from build123d import *

# Parameters (mm, degrees)
F0_R     = 2.5
F1_DEPTH = 5


with BuildPart() as f1:
    # F0 (on Front) → F1 (new body)
    with BuildSketch(Plane.XZ):
        with BuildLine():
            ThreePointArc((0, -4.25), (3.005204, -3.005204), (4.25, 0))
            ThreePointArc((4.25, 0), (3.005204, 3.005204), (0, 4.25))
            ThreePointArc((0, 4.25), (-4.25, 0), (0, -4.25))
        make_face()
        Circle(F0_R, mode=Mode.SUBTRACT)
        with BuildLine():
            ThreePointArc((30.75, 0), (29.505204, 3.005204), (26.5, 4.25))
            ThreePointArc((26.5, 4.25), (22.25, 0), (26.5, -4.25))
            ThreePointArc((26.5, -4.25), (29.505204, -3.005204), (30.75, 0))
        make_face()
        with Locations((26.5, 0)):
            Circle(F0_R, mode=Mode.SUBTRACT)
        with BuildLine():
            ThreePointArc((0, 4.25), (3.005204, 3.005204), (4.25, 0))
            ThreePointArc((4.25, 0), (3.005204, -3.005204), (0, -4.25))
            Line((0, -4.25), (26.5, -4.25))
            ThreePointArc((26.5, -4.25), (22.25, 0), (26.5, 4.25))
            Line((26.5, 4.25), (0, 4.25))
        make_face()
    extrude(amount=F1_DEPTH)


solid = f1.part
For this review, take the finished solid that the model builds, in its own axes (mm). Round coordinates to 2 decimals unless told otherwise and drop trailing zeros. Loops run counter-clockwise (first coordinate to the right, second up) from the corner with the lowest first, then second, coordinate; pieces in that order, holes last. Notation, with made-up numbers: (64, 41.5) - (119, 41.5) arc R10 ccw to (119, 58.5) - close; hole circle Ø1 at (-10, 50.5). An arc over 180 degrees is marked (long way). Answer as CSV lines item,"result".
(1) Insertion check: P1, Ø1.5, axis at y = -2, z = -2, coming from the +X side; P2, Ø1, axis at y = -3, z = 2.5, coming from the -X side. Each pin has a flat end and moves straight along its axis. Give the tip position at first contact, or say it passes through.
Checked values:
P1,"stops at x = 30.56"
P2,"stops at x = -3.75"
(2) Consider section C-C on y = -4.35. Give the boundary of the cut face in (x, z), then the cut area to 3 significant figures.
Checked values:
outline,"(0, -4.25) - (26.5, -4.25) arc R4.25 ccw to (30.75, 0) arc R4.25 ccw to (26.5, 4.25) - (0, 4.25) arc R4.25 ccw to start; hole circle Ø5 at (0, 0); hole circle Ø5 at (26.5, 0)"
area,"243 mm2"
(3) Consider section D-D on z = -3. Give the boundary of the cut face in (x, y), then the cut area to 3 significant figures.
Checked values:
outline,"(-3.01, -5) - (29.51, -5) - (29.51, 0) - (-3.01, 0) - close"
area,"163 mm2"
(4) Consider section A-A on z = 2. Give the boundary of the cut face in (x, y).
Checked values:
outline,"(-3.75, -5) - (-1.5, -5) - (-1.5, 0) - (-3.75, 0) - close; (1.5, -5) - (25, -5) - (25, 0) - (1.5, 0) - close; (28, -5) - (30.25, -5) - (30.25, 0) - (28, 0) - close"
(5) Mouldability with a two-part tool opening along X and no side actions: class faces 1 (the face through (24, -2, 0)), 2 (the face through (-4.25, -2.46, 0.09)), 3 (the face through (13, -2, -4.25)) as +X half, -X half, draft (parallel to the pull), parting line (faces both ways), or undercut.
Checked values:
face 1,"undercut"
face 2,"-X half"
face 3,"draft"
(6) Consider section B-B on x = 28.5. Give the boundary of the cut face in (y, z).
Checked values:
outline,"(-5, -3.75) - (0, -3.75) - (0, -1.5) - (-5, -1.5) - close; (-5, 1.5) - (0, 1.5) - (0, 3.75) - (-5, 3.75) - close"
(7) Wall thickness on line 1 (X direction, y = -3.05, z = -0.75); line 2 (X direction, y = -2.75, z = 1.5); line 3 (Z direction, x = 26.5, y = -1.6): over which ranges is each line inside the solid? List them lowest first.
Checked values:
line 1,"x = -4.18 to -2.38, 2.38 to 24.12, 28.88 to 30.68"
line 2,"x = -3.98 to -2, 2 to 24.5, 28.5 to 30.48"
line 3,"z = -4.25 to -2.5, 2.5 to 4.25"
